Work out the finished part from the listing and answer in its coordinate system (mm). A direction names the side the tool comes from. Give positions to 0.01 mm unless a question says otherwise; leave off trailing zeros. Loops run counter-clockwise (first coordinate to the right, second up) from the corner with the lowest first, then second, coordinate; pieces in that order, holes last. Notation, with made-up numbers: (61.5, 53) - (116.5, 53) arc R25 cw to (116.5, 90) - close; hole circle Ø11 at (4.5, -15.75). An arc over 180 degrees is marked (long way). One line per question, with ' | ' between items. Start each with the question number.
1. Section A-A (y = -116) is taken. Determine the outline of the cut face in (x, z).
2. Which of the six approach directions +Z, -Z, +X, -X, +Y, -Y give full straight-line access (tool end or side, diameter ignored) to faces 4 (the face through (-47.367, -12.386, 213.304)), 5 (the face through (-19.524, -377.488, 4.336)), 6 (the face through (-42.954, -399.035, 9.538))?
3. For a pull along X with two mould halves and no side action, classify faces 1 (the face through (-9, -401.5, -19)), 2 (the face through (93.455, -226.655, -29.43)), 3 (the face through (-214.28, -12.52, -47.58)) as released by +X, released by -X, zero draft, split by the parting line, or undercut.
4. Section B-B (y = -267) is taken. Determine the outline of the cut face in (x, z), plus the area to 3 significant figures.
5. Each of these flat-tipped pins is pushed along its axis until it touches: pin 1 (1 mm diameter, centred on x = 27.5, z = 14, fed in from +Y); pin 2 (1 mm diameter, centred on y = -106.5, z = 48.5, fed in from +X); pin 3 (3 mm diameter, centred on x = 5.5, z = -95, fed in from +Y); pin 4 (8 mm diameter, centred on x = -25.98, z = -15, fed in from -Y). Where does it stop, or does it pass through?
6. Find the intervals of material crossed by line 1 (X direction, y = -368, z = 0); line 2 (Z direction, x = -112, y = -122); line 3 (Z direction, x = 157, y = -52.5), in increasing order.
from build123d import *

# Parameters (mm, degrees)
CROQUIS1_R              = 219.5
SALIENTE_EXTRUIR1_DEPTH = 25.4
CROQUIS3_R              = 20
CROQUIS2_R              = 219.5
CROQUIS4_R              = 20
SALIENTE_EXTRUIR2_DEPTH = 40
CROQUIS10_R             = 44
SALIENTE_EXTRUIR6_DEPTH = 2.5
CROQUIS15_R             = 19
CORTAR_EXTRUIR1_DEPTH   = 504.560075947
CROQUIS16_R             = 3
CORTAR_EXTRUIR2_DEPTH   = 5


# Read off the part's stored shape, not the designer's step: Vaciado3
with BuildPart() as part:
    # Croquis1 → Saliente-Extruir1 (new body)
    with BuildSketch(Plane(origin=(0, 0, 0), x_dir=(1, 0, 0), z_dir=(0, 1, 0))):
        with Locations(Location((0, 0, 0), (0, 0, 270))):
            Circle(CROQUIS1_R)
    extrude(amount=-SALIENTE_EXTRUIR1_DEPTH)

    # Croquis3 → Recubrir1 section 0
    with BuildSketch(Plane(origin=(0, -359, 0), x_dir=(1, 0, 0), z_dir=(0, 1, 0))):
        Circle(CROQUIS3_R)
    # Croquis2 → Recubrir1 section 1
    with BuildSketch(Plane.XZ.offset(25.4)):
        Circle(CROQUIS2_R)
    loft()

    # Croquis4 → Saliente-Extruir2 (add)
    with BuildSketch(Plane.XZ.offset(359)):
        with Locations(Location((0, 0, 0), (0, 0, 270))):
            Circle(CROQUIS4_R)
    extrude(amount=SALIENTE_EXTRUIR2_DEPTH)

    # Vaciado3 outline → Vaciado3 (revolve, cut)
    with BuildSketch(Plane.XY):
        Polygon((218.5, -25.123799723), (218.5, 0), (0, 0), (0, -399), (19, -399), (19, -358.723799723), align=None)
    revolve(axis=Axis((0, 0, 0), (0, 1, 0)), mode=Mode.SUBTRACT)

    # Croquis10 → Saliente-Extruir6 (add, symmetric)
    with BuildSketch(Plane.XZ.offset(399)):
        with Locations(Location((0, 0, 0), (0, 0, 270))):
            Circle(CROQUIS10_R)
    extrude(amount=SALIENTE_EXTRUIR6_DEPTH, both=True)

    # Croquis15 → Cortar-Extruir1 (cut, through all)
    with BuildSketch(Plane(origin=(0, -396.5, 0), x_dir=(1, 0, 0), z_dir=(0, 1, 0))):
        with Locations(Location((0, 0, 0), (0, 0, 270))):
            Circle(CROQUIS15_R)
    extrude(amount=-CORTAR_EXTRUIR1_DEPTH, mode=Mode.SUBTRACT)

    # Croquis16 → Cortar-Extruir2 (cut)
    with BuildSketch(Plane.XZ.offset(401.5)):
        with Locations(Location((0, -30, 0), (0, 0, 270))):
            Circle(CROQUIS16_R)
        with Locations(Location((-25.980762114, -15, 0), (0, 0, 270))):
            Circle(CROQUIS16_R)
        with Locations(Location((-25.980762114, 15, 0), (0, 0, 270))):
            Circle(CROQUIS16_R)
        with Locations(Location((0, 30, 0), (0, 0, 270))):
            Circle(CROQUIS16_R)
        with Locations(Location((25.980762114, 15, 0), (0, 0, 270))):
            Circle(CROQUIS16_R)
        with Locations(Location((25.980762114, -15, 0), (0, 0, 270))):
            Circle(CROQUIS16_R)
    extrude(amount=-CORTAR_EXTRUIR2_DEPTH, mode=Mode.SUBTRACT)


solid = part.part
Conclusion:
1) outline: circle Ø330.64 at (0, 0); hole circle Ø328.31 at (0, 0)
2) face 4: +Y | face 5: none | face 6: -Y
3) face 1: zero draft | face 2: undercut | face 3: split by the parting line
4) outline: circle Ø150.04 at (0, 0); hole circle Ø147.71 at (0, 0) | area: 545 mm²
5) pin 1: y = -338.06 | pin 2: x = 164.32 | pin 3: y = -228.86 | pin 4: y = -401.5
6) line 1: -20 to -19, 19 to 20 | line 2: -116.67 to -115.05, 115.05 to 116.67 | line 3: -129.15 to -127.31, 127.31 to 129.15
